Source: three-view drawing plus pictorial views. Frame: mm from the lowest corner of the part. Give positions to 0.01 mm unless a question says otherwise; leave off trailing zeros. Order: outer loops, then holes, each group sorted by start corner. A loop starts at its lowest first (then second) coordinate and runs counter-clockwise, first axis right, second up. Notation, with made-up numbers: (-27, 26) -> (-2, 26) arc R26 cw to (-2, 44) -> close; hole circle Ø1 at (10, 68.25). An arc over 180 degrees is marked (long way). Write item = value, one per line.
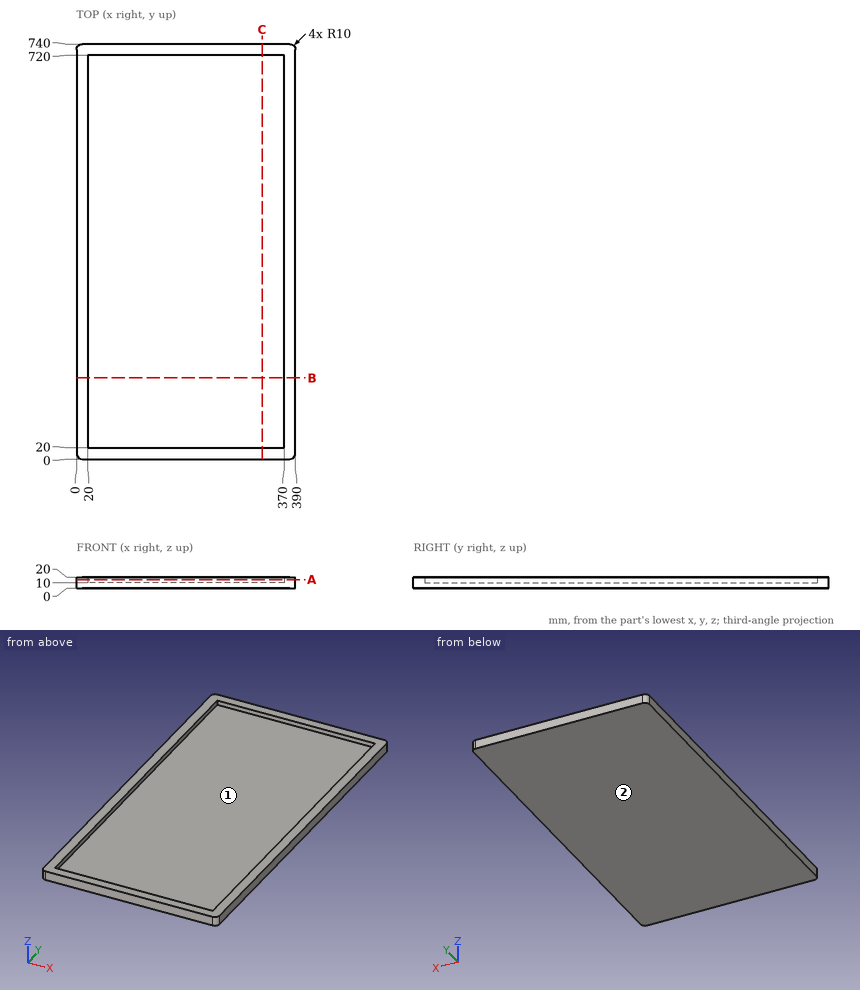
1) Line query: line 1 (Y direction, x = 139, z = 15.25); line 2 (X direction, y = 212.5, z = 15.75); line 3 (Z direction, x = 130.5, y = 626). Output: solid intervals per line, ascending. Write a range as from..to.
Check sheet entries:
line_1 = 0..20, 720..740
line_2 = 0..20, 370..390
line_3 = 0..10
2) Section query A-A (z = 15.75). Output: boundary loops of the cut face in (x, y), plus the area to 3 significant figures.
Check sheet entries:
outline = (0, 10) arc R10 ccw to (10, 0) -> (380, 0) arc R10 ccw to (390, 10) -> (390, 730) arc R10 ccw to (380, 740) -> (10, 740) arc R10 ccw to (0, 730) -> close; hole (20, 20) -> (370, 20) -> (370, 720) -> (20, 720) -> close
area = 43,500 mm²
3) Section query C-C (x = 331). Output: boundary loops of the cut face in (y, z), plus the area to 3 significant figures.
Check sheet entries:
outline = (0, 0) -> (740, 0) -> (740, 20) -> (720, 20) -> (720, 10) -> (20, 10) -> (20, 20) -> (0, 20) -> close
area = 7,800 mm²
4) Mould query, pull axis X, two halves, no side actions, for the marked faces 1 and 2. Classes: +X half, -X half, draft (parallel to the pull), parting line (faces both ways), or undercut.
Check sheet entries:
face_1 = undercut
face_2 = draft
5) Section query B-B (y = 145). Output: boundary loops of the cut face in (x, z).
Check sheet entries:
outline = (0, 0) -> (390, 0) -> (390, 20) -> (370, 20) -> (370, 10) -> (20, 10) -> (20, 20) -> (0, 20) -> close
6) First-contact query: P1, Ø6, axis at x = 110.5, y = 184.5, coming from the +Z side. Flat tip, straight axial feed; report the tip coordinate or a pass-through.
Check sheet entries:
P1 = 10
